Geometry: see drawing. Coordinates: mm, zero at the bounding-box minimum. Give positions to 0.01 mm unless a question says otherwise; leave off trailing zeros. Write each loop counter-clockwise with the first axis right and the second up, starting at its lowest first coordinate (ties: lowest second). Pieces come first, ordered by that corner, then holes.
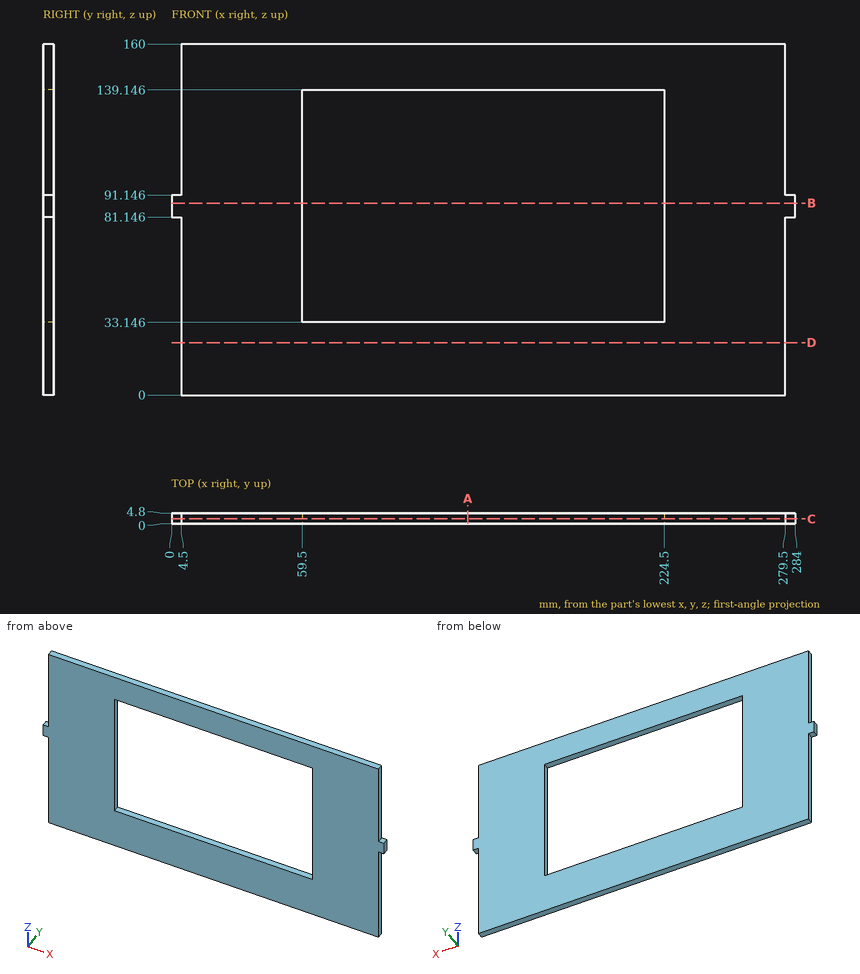
Q1. Section A-A, the plane x = 135. Return the cut outline in (y, z) (1 decimal), then the cut area to 3 significant figures.
Q2. Section B-B, the plane z = 87.5. Return the cut outline in (x, y).
Q3. Section D-D, the plane z = 24. Return the cut outline in (x, y).
Q4. Pin query (flat end, axial travel): pin 1 (2.5 mm diameter, centred on y = 3, z = 37, fed in from -X); pin 2 (1.4 mm diameter, centred on y = 2, z = 40.5, fed in from +X). Return the tip coordinate at first contact, or that it passes through.
Q5. Material intervals for line 1 along Z through (x, y) = (173, 0.3) (1 decimal); line 2 along X through (y, z) = (4.15, 71.5); line 3 along X through (y, z) = (3.55, 89), sorted ascending.
Q6. Section C-C, the plane y = 2.2. Return the cut outline in (x, z) (1 decimal), then the cut area to 3 significant figures.
Solutions:
1. outline: (0, 0) - (4.8, 0) - (4.8, 33.1) - (0, 33.1) - close; (0, 139.1) - (4.8, 139.1) - (4.8, 160) - (0, 160) - close
1. area: 259 mm2
2. outline: (0, 0) - (59.5, 0) - (59.5, 4.8) - (0, 4.8) - close; (224.5, 0) - (284, 0) - (284, 4.8) - (224.5, 4.8) - close
3. outline: (4.5, 0) - (279.5, 0) - (279.5, 4.8) - (4.5, 4.8) - close
4. pin 1: stops at x = 4.5
4. pin 2: stops at x = 279.5
5. line 1: z = 0 to 33.1, 139.1 to 160
5. line 2: x = 4.5 to 59.5, 224.5 to 279.5
5. line 3: x = 0 to 59.5, 224.5 to 284
6. outline: (0, 81.1) - (4.5, 81.1) - (4.5, 0) - (279.5, 0) - (279.5, 81.1) - (284, 81.1) - (284, 91.1) - (279.5, 91.1) - (279.5, 160) - (4.5, 160) - (4.5, 91.1) - (0, 91.1) - close; hole (59.5, 33.1) - (224.5, 33.1) - (224.5, 139.1) - (59.5, 139.1) - close
6. area: 26,600 mm2
